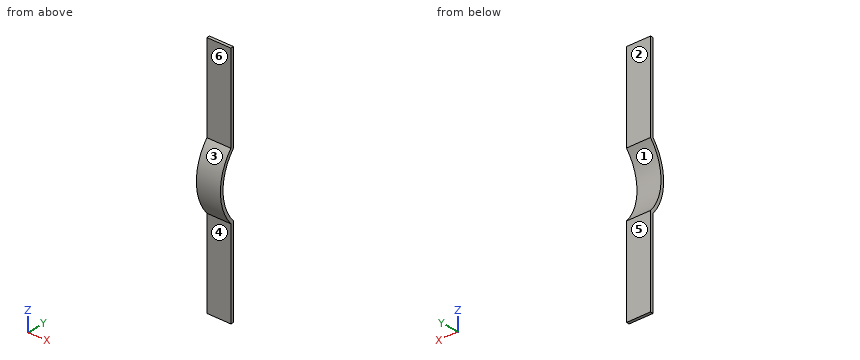
```python
from build123d import *

# Parameters (mm, degrees)
BOSS_EXTRUDE1_DEPTH      = 25.4
BOSS_EXTRUDE2_REACH      = 350.576
BOSS_EXTRUDE2_END_RADIUS = 107.95
SKETCH2_W                = 50.8
SKETCH2_H                = 6.35


with BuildPart() as part:
    # Sketch1 → Boss-Extrude1 (new, symmetric)
    with BuildSketch(Plane(origin=(0, 0, 0), x_dir=(0, 0, -1), z_dir=(1, 0, 0))):
        with BuildLine():
            Line((-76.464125575, -76.2), (-67.202083301, -76.2))
            ThreePointArc((-67.202083301, -76.2), (0, -101.6), (67.202083301, -76.2))
            Line((67.202083301, -76.2), (76.464125575, -76.2))
            ThreePointArc((76.464125575, -76.2), (0, -107.95), (-76.464125575, -76.2))
        make_face()
    extrude(amount=BOSS_EXTRUDE1_DEPTH, both=True)

    # Boss-Extrude2: up to this cylinder (the profile starts outside it)
    boss_extrude2_end = Plane(origin=(0, 0, 0), z_dir=(-1, 0, 0)) * Cylinder(BOSS_EXTRUDE2_END_RADIUS, 918.052, mode=Mode.PRIVATE)
    # Sketch2 → Boss-Extrude2 (add, up to the surface)
    with BuildSketch(Plane.XY.offset(254), mode=Mode.PRIVATE) as boss_extrude2_sk1:
        with Locations((0, -79.375)):
            Rectangle(SKETCH2_W, SKETCH2_H)
    boss_extrude2_tool1 = extrude(boss_extrude2_sk1.sketch, amount=-BOSS_EXTRUDE2_REACH, mode=Mode.PRIVATE) - boss_extrude2_end
    boss_extrude2 = boss_extrude2_tool1.solids().sort_by_distance((0, -79.375, 254))[0]
    add(boss_extrude2)

    # Mirror1: Boss-Extrude2 across plane
    add(boss_extrude2.mirror(Plane.XY))


solid = part.part
```
Geometry: final body of the model. Coordinates: model frame, mm. Face numbers are marked on the shaded views. A direction names the side the tool comes from. Coordinates: 2 decimals unless noted, no trailing zeros. Order: outer loops, then holes, each group sorted by start corner. A loop starts at its lowest first (then second) coordinate and runs counter-clockwise, first axis right, second up. Notation, with made-up numbers: M 29,-7.5 L 85,-7.5 A15 cw 85,0.5 Z; hole C 24.25,17.25 d7. An arc over 180 degrees is marked long. Answer as CSV lines item,"result".
Q1. Draft query along Z for the marked faces 1, 2 and 3. Return one class per face: pulls with the +Z half, pulls with the -Z half, needs draft (parallel to the pull), parting line crosses it, or undercut.
Answers:
face 1,"undercut"
face 2,"needs draft"
face 3,"parting line crosses it"
Q2. Section C-C on z = -152.5. Return the cut outline in (x, y), and give its area (3 significant figures).
Answers:
outline,"M -25.4,-82.55 L 25.4,-82.55 L 25.4,-76.2 L -25.4,-76.2 Z"
area,"323 mm^2"
Q3. Set-up query: the marked faces 4, 5 and 6. Return all of +Z, -Z, +X, -X, +Y, -Y with unobstructed straight access to the full face (end or side cutting, diameter ignored); none if empty.
Answers:
face 4,"-Z, +X, -X, -Y"
face 5,"+Z, -Z, +X, -X, +Y"
face 6,"+Z, +X, -X, -Y"
Q4. Section B-B on y = -93.5. Return the cut outline in (x, z).
Answers:
outline,"M -25.4,-53.95 L 25.4,-53.95 L 25.4,-39.75 L -25.4,-39.75 Z; M -25.4,39.75 L 25.4,39.75 L 25.4,53.95 L -25.4,53.95 Z"
Q5. Line query: probe 1 along Y at (x, z) = (5.5, 73.5); probe 2 along Z at (x, y) = (7, -92.5); probe 3 along Z at (x, y) = (-20, -94.5). Output: solid intervals per line, ascending. Write a range as [from, to].
Answers:
probe 1,"y = [-82.55, -76.2]"
probe 2,"z = [-55.65, -42.03], [42.03, 55.65]"
probe 3,"z = [-52.18, -37.31], [37.31, 52.18]"
Q6. First-contact query: P1, Ø6, axis at x = -7, z = 167.5, coming from the -Y side; P2, Ø1.5, axis at x = 12, z = 63.5, coming from the +Y side; P3, Ø12, axis at x = 9, y = -92.5, coming from the +Z side. Flat tips, straight axial feed; report the tip coordinate or a pass-through.
Answers:
P1,"stops at y = -82.55"
P2,"stops at y = -78.71"
P3,"stops at z = 64.58"
Q7. Section D-D on z = 36. Return the cut outline in (x, y).
Answers:
outline,"M -25.4,-101.77 L 25.4,-101.77 L 25.4,-95.01 L -25.4,-95.01 Z"
Q8. Section A-A on x = -4. Return the cut outline in (y, z), and give its area (3 significant figures).
Answers:
outline,"M -82.55,-254 L -76.2,-254 L -76.2,-67.2 A101.6 cw -76.2,67.2 L -76.2,254 L -82.55,254 L -82.55,69.56 A107.95 ccw -82.55,-69.56 Z"
area,"3,300 mm^2"
